The model under review builds one solid part; all positions refer to its coordinate system, in mm. Give positions to 0.01 mm unless a question says otherwise; leave off trailing zeros. Loops run counter-clockwise (first coordinate to the right, second up) from the corner with the lowest first, then second, coordinate; pieces in that order, holes last. Notation, with made-up numbers: M 18,-16 L 69,-16 A14 cw 69,10 Z; hole C 8.25,58 d3. An arc over 180 degrees is marked long. One line per item, written item: value. Start each with the question number.
Q1. We need section D-D on x = -11. Write out the cut boundary in (y, z), plus the area to 3 significant figures.
Q2. We need section A-A on x = 1. Write out the cut boundary in (y, z).
Q3. For pin 1 (1.8 mm diameter, centred on x = 4.2, y = 5.2, fed in from +Z); pin 2 (1.5 mm diameter, centred on x = -21, z = -29.5, fed in from +Y); pin 3 (2 mm diameter, centred on x = 24.5, z = 34.5, fed in from +Y); pin 4 (0.6 mm diameter, centred on x = -17.5, y = 1.5, fed in from -Z), all flat-tipped, find the tip position at first contact; note any pin that passes through.
Q4. To check wall thickness, follow line 1 along Y through (x, z) = (4.2, 44.8); line 2 along Z through (x, y) = (1.5, 6); line 3 along Z through (x, y) = (-23, 1). State the ranges of each line that lie inside material, in increasing order. Write a range as from..to.
Q5. We need section C-C on z = 4.5. Write out the cut boundary in (x, y), plus the area to 3 significant figures.
Q6. We need section B-B on y = 1. Write out the cut boundary in (x, z).
```python
from build123d import *

# Parameters (mm, degrees)
SKETCH1_W           = 60
SKETCH1_H           = 84
BOSS_EXTRUDE1_DEPTH = 2
SKETCH4_W           = 2
SKETCH4_H           = 2
BOSS_EXTRUDE3_DEPTH = 4
SKETCH5_W           = 12.4
SKETCH5_H           = 2
SKETCH5_R           = 2
SKETCH5_R_2         = 1
BOSS_EXTRUDE4_DEPTH = 4


with BuildPart() as part:
    # Sketch1 → Boss-Extrude1 (new body)
    with BuildSketch(Plane(origin=(0, 0, 0), x_dir=(1, 0, 0), z_dir=(0, 1, 0))):
        Rectangle(SKETCH1_W, SKETCH1_H)
    extrude(amount=BOSS_EXTRUDE1_DEPTH)

    # Sketch4 → Boss-Extrude3 (add)
    with BuildSketch(Plane(origin=(0, 2, 0), x_dir=(1, 0, 0), z_dir=(0, 1, 0))):
        with Locations((-24.7, 34.7)):
            Rectangle(SKETCH4_W, SKETCH4_H)
        with Locations((24.7, 34.7)):
            Rectangle(SKETCH4_W, SKETCH4_H)
        with Locations((24.7, -34.7)):
            Rectangle(SKETCH4_W, SKETCH4_H)
        with Locations((-24.7, -34.7)):
            Rectangle(SKETCH4_W, SKETCH4_H)
    extrude(amount=BOSS_EXTRUDE3_DEPTH)

    # Sketch5 → Boss-Extrude4 (add)
    # profile 1 of 4: a face of its own
    with BuildSketch(Plane(origin=(0, 0, -42), x_dir=(-1, 0, 0), z_dir=(0, 0, -1))):
        with Locations((0, 1)):
            Rectangle(SKETCH5_W, SKETCH5_H)
    # profile 2 of 4: a face of its own
    with BuildSketch(Plane(origin=(0, 0, -42), x_dir=(-1, 0, 0), z_dir=(0, 0, -1))):
        with BuildLine():
            ThreePointArc((-2.2, 5.2), (-4.2, 3.2), (-6.2, 5.2))
            Line((-6.2, 5.2), (-6.2, 2))
            Line((-6.2, 2), (6.2, 2))
            Line((6.2, 2), (6.2, 5.2))
            ThreePointArc((6.2, 5.2), (2.785786438, 3.785786438), (4.2, 7.2))
            Line((4.2, 7.2), (-4.2, 7.2))
            ThreePointArc((-4.2, 7.2), (-2.785786438, 6.614213562), (-2.2, 5.2))
        make_face()
    # profile 3 of 4: a face of its own
    with BuildSketch(Plane(origin=(0, 0, -42), x_dir=(-1, 0, 0), z_dir=(0, 0, -1))):
        with Locations((-4.2, 5.2)):
            Circle(SKETCH5_R)
        with Locations((-4.2, 5.2)):
            Circle(SKETCH5_R_2, mode=Mode.SUBTRACT)
    # profile 4 of 4: a face of its own
    with BuildSketch(Plane(origin=(0, 0, -42), x_dir=(-1, 0, 0), z_dir=(0, 0, -1))):
        with Locations((4.2, 5.2)):
            Circle(SKETCH5_R)
        with Locations((4.2, 5.2)):
            Circle(SKETCH5_R_2, mode=Mode.SUBTRACT)
    boss_extrude4 = extrude(amount=BOSS_EXTRUDE4_DEPTH)

    # Mirror1: Boss-Extrude4 across plane
    add(boss_extrude4.mirror(Plane.XY))


solid = part.part
```
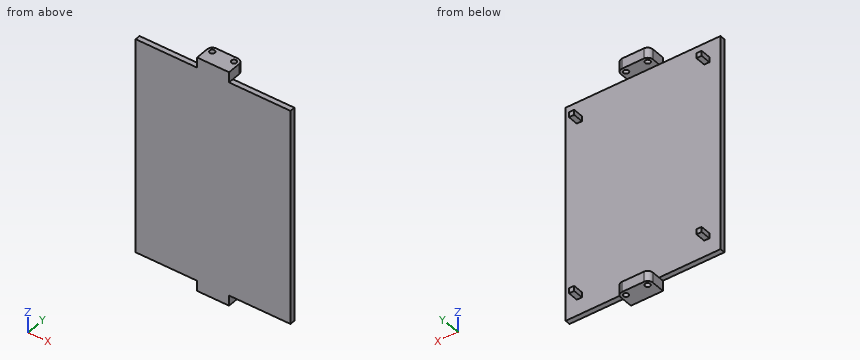
Solved:
1. outline: M 0,-42 L 2,-42 L 2,42 L 0,42 Z
1. area: 168 mm2
2. outline: M 0,-46 L 7.2,-46 L 7.2,-42 L 2,-42 L 2,42 L 7.2,42 L 7.2,46 L 0,46 Z
3. pin 1: through
3. pin 2: y = 2
3. pin 3: y = 6
3. pin 4: z = -42
4. line 1: 0..4.2, 6.2..7.2
4. line 2: -46..-42, 42..46
4. line 3: -42..42
5. outline: M -30,0 L 30,0 L 30,2 L -30,2 Z
5. area: 120 mm2
6. outline: M -30,-42 L -6.2,-42 L -6.2,-46 L 6.2,-46 L 6.2,-42 L 30,-42 L 30,42 L 6.2,42 L 6.2,46 L -6.2,46 L -6.2,42 L -30,42 Z
